from build123d import *

# Parameters (mm, degrees)
SKETCH1_W               = 457.2
SKETCH1_H               = 635
BOSS_EXTRUDE1_DEPTH     = 7.62
SKETCH2_W               = 12.7
SKETCH2_H               = 254
CUT_EXTRUDE1_DEPTH      = 392.308413403
SKETCH5_W               = 25.4
SKETCH5_H               = 25.4
BOSS_EXTRUDE3_DEPTH     = 228.6
SKETCH6_R               = 6.35
BOSS_EXTRUDE4_DEPTH     = 50.8
BOSS_EXTRUDE6_DEPTH     = 38.1
CUT_EXTRUDE2_DEPTH      = 426.395026299
CUT_EXTRUDE2_DEPTH_BACK = 38.1
SKETCH8_W               = 152.4
SKETCH8_H               = 38.1
BOSS_EXTRUDE7_DEPTH     = 2.54
SKETCH9_W               = 457.2
SKETCH9_H               = 38.1
CUT_EXTRUDE3_DEPTH      = 10.16
CUT_EXTRUDE4_DEPTH      = 601.268156743
CUT_EXTRUDE4_DEPTH_BACK = 601.268156743
SKETCH10_R              = 6.35
SKETCH11_R              = 5.08
CUT_EXTRUDE5_DEPTH      = 25.4
SKETCH12_W              = 67.801888186
SKETCH12_H              = 38.1
CUT_EXTRUDE7_DEPTH      = 599.120114693
SKETCH16_R              = 7.5
CUT_EXTRUDE9_DEPTH      = 425.643638831
LPATTERN1_COUNT         = 5
LPATTERN1_PITCH         = 50
LPATTERN2_COUNT         = 3
LPATTERN2_PITCH         = 50


with BuildPart() as part:
    # Sketch1 → Boss-Extrude1 (new body)
    with BuildSketch(Plane(origin=(0, 0, 0), x_dir=(1, 0, 0), z_dir=(0, 1, 0))):
        Rectangle(SKETCH1_W, SKETCH1_H)
    extrude(amount=BOSS_EXTRUDE1_DEPTH)

    # Sketch2 → Cut-Extrude1 (cut, through all)
    with BuildSketch(Plane(origin=(0, 7.62, 0), x_dir=(1, 0, 0), z_dir=(0, 1, 0))):
        with Locations((-95.25, 152.4)):
            Rectangle(SKETCH2_W, SKETCH2_H)
        with Locations((-95.25, -152.4)):
            Rectangle(SKETCH2_W, SKETCH2_H)
        with Locations((-184.15, 152.4)):
            Rectangle(SKETCH2_W, SKETCH2_H)
        with Locations((-184.15, -152.4)):
            Rectangle(SKETCH2_W, SKETCH2_H)
        with Locations((184.15, 152.4)):
            Rectangle(SKETCH2_W, SKETCH2_H)
        with Locations((95.25, 152.4)):
            Rectangle(SKETCH2_W, SKETCH2_H)
        with Locations((184.15, -152.4)):
            Rectangle(SKETCH2_W, SKETCH2_H)
        with Locations((95.25, -152.4)):
            Rectangle(SKETCH2_W, SKETCH2_H)
    extrude(amount=-CUT_EXTRUDE1_DEPTH, mode=Mode.SUBTRACT)

    # Sketch5 → Boss-Extrude3 (add)
    with BuildSketch(Plane(origin=(228.6, 0, 0), x_dir=(0, 0, -1), z_dir=(1, 0, 0))):
        with Locations((139.7, -12.7)):
            Rectangle(SKETCH5_W, SKETCH5_H)
    boss_extrude3 = extrude(amount=-BOSS_EXTRUDE3_DEPTH)

    # Sketch6 → Boss-Extrude4 (add)
    with BuildSketch(Plane(origin=(228.6, 0, 0), x_dir=(0, 0, -1), z_dir=(1, 0, 0))):
        with Locations(Location((139.7, -12.7, 0), (0, 0, 180))):
            Circle(SKETCH6_R)
    boss_extrude4 = extrude(amount=BOSS_EXTRUDE4_DEPTH)

    # Sketch3 → Boss-Extrude6 (add)
    with BuildSketch(Plane.XZ):
        Polygon((-228.6, 292.1), (228.6, 292.1), (228.6, -5.532066332), (-228.6, 215.9), align=None)
    extrude(amount=BOSS_EXTRUDE6_DEPTH)

    # Mirror2: Boss-Extrude3, Boss-Extrude4 across plane
    add(boss_extrude3.mirror(Plane(origin=(0, 0, 0), x_dir=(0, 0, 1), z_dir=(1, 0, 0))))
    add(boss_extrude4.mirror(Plane(origin=(0, 0, 0), x_dir=(0, 0, 1), z_dir=(1, 0, 0))))

    # Sketch7 → Cut-Extrude2 (cut, two sides: drawn at the far end of the back side and taken through both)
    with BuildSketch(Plane.XZ.offset(38.1).offset(-CUT_EXTRUDE2_DEPTH_BACK)):
        Polygon((-226.06, 214.669821854), (226.06, -4.301888186), (226.06, 289.56), (-226.06, 289.56), align=None)
    extrude(amount=CUT_EXTRUDE2_DEPTH + CUT_EXTRUDE2_DEPTH_BACK, mode=Mode.SUBTRACT)

    # Sketch8 → Boss-Extrude7 (add)
    with BuildSketch(Plane.ZY.offset(228.6)):
        with Locations((139.7, -19.05)):
            Rectangle(SKETCH8_W, SKETCH8_H)
    extrude(amount=-BOSS_EXTRUDE7_DEPTH)

    # Sketch9 → Cut-Extrude3 (cut)
    with BuildSketch(Plane.XY.offset(292.1)):
        with Locations((0, -19.05)):
            Rectangle(SKETCH9_W, SKETCH9_H)
    extrude(amount=-CUT_EXTRUDE3_DEPTH, mode=Mode.SUBTRACT)

    # Sketch10 → Cut-Extrude4 (cut, two sides: drawn at the far end of the back side and taken through both)
    with BuildSketch(Plane.ZY.offset(228.6).offset(-CUT_EXTRUDE4_DEPTH_BACK)):
        with Locations((255.61861162, -25.709236818)):
            Circle(SKETCH10_R)
    extrude(amount=CUT_EXTRUDE4_DEPTH + CUT_EXTRUDE4_DEPTH_BACK, mode=Mode.SUBTRACT)

    # Sketch11 → Cut-Extrude5 (cut)
    with BuildSketch(Plane(origin=(279.4, 0, 0), x_dir=(0, 0, -1), z_dir=(1, 0, 0))):
        with Locations((139.7, -12.7)):
            Circle(SKETCH11_R)
    cut_extrude5 = extrude(amount=-CUT_EXTRUDE5_DEPTH, mode=Mode.SUBTRACT)

    # Mirror3: Cut-Extrude5 across plane
    add(cut_extrude5.mirror(Plane(origin=(0, 0, 0), x_dir=(0, 0, 1), z_dir=(1, 0, 0))), mode=Mode.SUBTRACT)

    # Sketch12 → Cut-Extrude7 (cut, through all)
    with BuildSketch(Plane.ZY.offset(-226.06)):
        with Locations((28.368877761, -19.05)):
            Rectangle(SKETCH12_W, SKETCH12_H)
    extrude(amount=-CUT_EXTRUDE7_DEPTH, mode=Mode.SUBTRACT)

    # Sketch16 → Cut-Extrude9 (cut, through all)
    with BuildSketch(Plane.XZ):
        with Locations(Location((0, -229.727054267, 0), (0, 0, 270))):
            Circle(SKETCH16_R)
    cut_extrude9 = extrude(amount=-CUT_EXTRUDE9_DEPTH, mode=Mode.SUBTRACT)

    # LPattern1: Cut-Extrude9 ×5
    with Locations(*[(0, 0, i * LPATTERN1_PITCH) for i in range(1, LPATTERN1_COUNT)]):
        add(cut_extrude9, mode=Mode.SUBTRACT)

    # LPattern2: Cut-Extrude9 ×3
    with Locations(*[(0, 0, -i * LPATTERN2_PITCH) for i in range(1, LPATTERN2_COUNT)]):
        add(cut_extrude9, mode=Mode.SUBTRACT)


solid = part.part
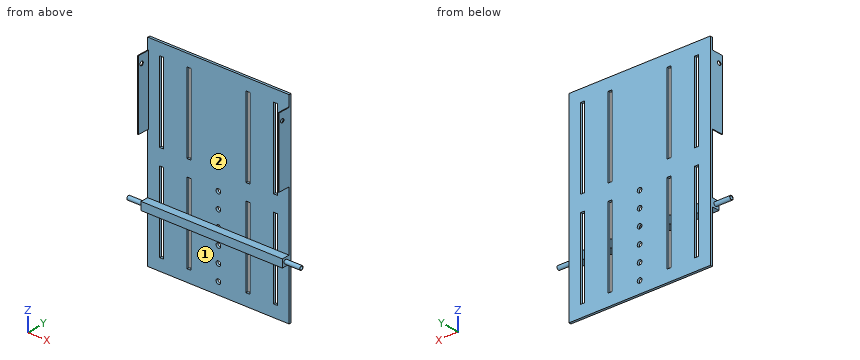
Verification items for the finished model (mm, model axes). Face numbers are marked on the shaded views. Coordinates: 2 decimals unless noted, no trailing zeros. Write each loop counter-clockwise with the first axis right and the second up, starting at its lowest first coordinate (ties: lowest second). Pieces come first, ordered by that corner, then holes. Notation, with made-up numbers: (5.5, 18) - (56.5, 18) arc R21 ccw to (56.5, 56) - close; hole circle Ø10 at (68.25, -3.75). An arc over 180 degrees is marked (long way). Answer as a JSON object with one key per item and string values.
(1) Cross-section at A-A on x = 0. Give the number of separate pieces and of enclosed holes in the cut face, plus the area to 3 significant figures.
Report:
{"separate pieces": "7", "enclosed holes": "0", "area": "4,800 mm^2"}
(2) Mould release check, pull along X, two halves, no side actions. Record for the marked faces 1 and 2: pulls with the +X half, pulls with the -X half, needs draft (parallel to the pull), parting line crosses it, or undercut.
Report:
{"face 1": "needs draft", "face 2": "undercut"}
(3) Gauge pin test, flat ends, axial feed: pin 1 Ø8.5 at (y, z) = (5.5, 133.5) entering from -X; pin 2 Ø1 at (x, y) = (10.5, -13) entering from +Z; pin 3 Ø6 at (x, z) = (-183, -150.5) entering from -Y; pin 4 Ø8 at (y, z) = (-13.5, -141) entering from -X. Record the tip position at first contact, or that the pin passes through.
Report:
{"pin 1": "x = -228.6", "pin 2": "z = -127", "pin 3": "y = -25.4", "pin 4": "x = -279.4"}
(4) Cross-section at D-D on x = 240. Record the cut outline in (y, z), plus the area to 3 significant figures.
Report:
{"outline": "circle Ø12.7 at (-12.7, -139.7)", "area": "127 mm^2"}
(5) Cross-section at B-B on z = 156. Record the cut outline in (x, y), plus the area to 3 significant figures.
Report:
{"outline": "(-228.6, -38.1) - (-226.06, -38.1) - (-226.06, 0) - (-190.5, 0) - (-190.5, 7.62) - (-228.6, 7.62) - close; (-177.8, 0) - (-101.6, 0) - (-101.6, 7.62) - (-177.8, 7.62) - close; (-88.9, 0) - (88.9, 0) - (88.9, 7.62) - (-88.9, 7.62) - close; (101.6, 0) - (177.8, 0) - (177.8, 7.62) - (101.6, 7.62) - close; (190.5, 0) - (226.06, 0) - (226.06, -38.1) - (228.6, -38.1) - (228.6, 7.62) - (190.5, 7.62) - close", "area": "3,290 mm^2"}
(6) Cross-section at C-C on x = 79.5. Record the cut outline in (y, z), plus the area to 3 significant figures.
Report:
{"outline": "(-25.4, -152.4) - (0, -152.4) - (0, -317.5) - (7.62, -317.5) - (7.62, 317.5) - (0, 317.5) - (0, -127) - (-25.4, -127) - close", "area": "5,480 mm^2"}
(7) Thickness scan on line 1 along Z through (x, y) = (-269, -12); line 2 along X through (y, z) = (-35, 273); line 3 along X through (y, z) = (2.5, 199.5). Record the ranges inside material, lowest first.
Report:
{"line 1": "-146.01 to -144.73, -134.67 to -133.39", "line 2": "-228.6 to -226.06, 226.06 to 228.6", "line 3": "-228.6 to -190.5, -177.8 to -101.6, -88.9 to 88.9, 101.6 to 177.8, 190.5 to 228.6"}
